Could you check a few things on this model? Use its own coordinates, in mm. A direction names the side the tool comes from. Give positions to 0.01 mm unless a question says otherwise; leave off trailing zeros. Write each loop counter-clockwise with the first axis right and the second up, starting at its lowest first coordinate (ties: lowest second). Pieces come first, ordered by that corner, then holes. Notation, with made-up numbers: (54, 64.25) -> (62, 64.25) arc R22 cw to (62, 101.25) -> close; hole circle Ø5 at (-35.5, 51.25). An arc over 180 degrees is marked (long way). One line per question, with ' | ' between items.
from build123d import *

# Parameters (mm, degrees)
SKETCH_1_R          = 1.85
EXTRUDE_1_DEPTH     = 13
SKETCH_2_R          = 2.6
CUT_EXTRUDE_1_DEPTH = 10
SKETCH_3_R          = 2.6
CUT_EXTRUDE_2_DEPTH = 10
FILLET_1_R          = 2
FILLET_2_R          = 1
SKETCH_4_R          = 3.5
SKETCH_4_R_2        = 1.85
CUT_EXTRUDE_3_DEPTH = 7
CUT_EXTRUDE_5_DEPTH = 61.729236251
CUT_EXTRUDE_START   = -4
SKETCH_6_R          = 5.5
SKETCH_6_R_2        = 2.6
CUT_EXTRUDE_6_DEPTH = 4
SKETCH_7_R          = 5.5
SKETCH_7_R_2        = 2.6
CUT_EXTRUDE_7_DEPTH = 4


with BuildPart() as part:
    # 草图1 → 凸台-拉伸1 (new body)
    with BuildSketch(Plane(origin=(0, 0, 0), x_dir=(1, 0, 0), z_dir=(0, 1, 0))):
        with BuildLine():
            ThreePointArc((-18.308849916, -29.829281164), (-22.856098901, -26.50657924), (-26.811555509, -22.497566339))
            Line((-26.811555509, -22.497566339), (-36.387111048, -30.53241146))
            ThreePointArc((-36.387111048, -30.53241146), (0, -47.5), (36.387111048, -30.53241146))
            Line((36.387111048, -30.53241146), (26.811555509, -22.497566339))
            ThreePointArc((26.811555509, -22.497566339), (22.856098901, -26.50657924), (18.308849916, -29.829281164))
            Line((18.308849916, -29.829281164), (19.814649575, -33.464603124))
            Line((19.814649575, -33.464603124), (9.651974717, -37.67412088))
            Line((9.651974717, -37.67412088), (8.146175058, -34.03879892))
            ThreePointArc((8.146175058, -34.03879892), (0, -35), (-8.146175058, -34.03879892))
            Line((-8.146175058, -34.03879892), (-9.651974717, -37.67412088))
            Line((-9.651974717, -37.67412088), (-19.814649575, -33.464603124))
            Line((-19.814649575, -33.464603124), (-18.308849916, -29.829281164))
        make_face()
        with BuildLine():
            ThreePointArc((-28.2020382, -30.0520382), (-28.237585432, -30.412955296), (-28.342861065, -30.76000255))
            ThreePointArc((-28.342861065, -30.76000255), (-31.866490969, -29.691121105), (-28.2020382, -30.0520382))
        make_face(mode=Mode.SUBTRACT)
        with BuildLine():
            ThreePointArc((1.85, -42.5), (-0.360917096, -44.314452769), (-1.709177135, -41.79203565))
            ThreePointArc((-1.709177135, -41.79203565), (0.360917096, -40.685547231), (1.85, -42.5))
        make_face(mode=Mode.SUBTRACT)
        with Locations(Location((30.0520382, -30.0520382, 0), (0, 0, 90))):
            Circle(SKETCH_1_R, mode=Mode.SUBTRACT)
    extrude(amount=EXTRUDE_1_DEPTH)

    # 草图2 → 切除-拉伸1 (cut)
    with BuildSketch(Plane(origin=(-14.733312146, 0, 35.569362002), x_dir=(-0.9238795325112864, 0, -0.38268343236509067), z_dir=(0.38268343236509067, 0, -0.9238795325112864))):
        with Locations((0, 6.5)):
            Circle(SKETCH_2_R)
    extrude(amount=-CUT_EXTRUDE_1_DEPTH, mode=Mode.SUBTRACT)

    # 草图3 → 切除-拉伸2 (cut)
    with BuildSketch(Plane(origin=(14.733312146, 0, 35.569362002), x_dir=(-0.9238795325112864, 0, 0.38268343236509067), z_dir=(-0.38268343236509067, 0, -0.9238795325112864))):
        with Locations((0, 6.5)):
            Circle(SKETCH_3_R)
    extrude(amount=-CUT_EXTRUDE_2_DEPTH, mode=Mode.SUBTRACT)

    # 圆角1
    fillet_1_edges = [part.edges().sort_by_distance(p)[0] for p in [
        (-26.811555509, 6.5, 22.497566339),
        (26.811555509, 6.5, 22.497566339),
        (36.387111048, 6.5, 30.53241146),
        (-36.387111048, 6.5, 30.53241146),
    ]]
    fillet(fillet_1_edges, radius=FILLET_1_R)

    # 圆角2
    fillet_2_edges = [part.edges().sort_by_distance(p)[0] for p in [
        (-18.308849916, 6.5, 29.829281164),
        (-8.146175058, 6.5, 34.03879892),
        (8.146175058, 6.5, 34.03879892),
        (18.308849916, 6.5, 29.829281164),
    ]]
    fillet(fillet_2_edges, radius=FILLET_2_R)

    # 草图4 → 切除-拉伸3 (cut)
    # profile 1 of 3: a face of its own
    with BuildSketch(Plane.XZ):
        with Locations(Location((-30.0520382, 30.0520382, 0), (0, 0, 270))):
            Circle(SKETCH_4_R)
        with Locations(Location((-30.0520382, 30.0520382, 0), (0, 0, 270))):
            Circle(SKETCH_4_R_2, mode=Mode.SUBTRACT)
    # profile 2 of 3: a face of its own
    with BuildSketch(Plane.XZ):
        with Locations(Location((0, 42.5, 0), (0, 0, 270))):
            Circle(SKETCH_4_R)
        with Locations(Location((0, 42.5, 0), (0, 0, 270))):
            Circle(SKETCH_4_R_2, mode=Mode.SUBTRACT)
    # profile 3 of 3: a face of its own
    with BuildSketch(Plane.XZ):
        with Locations(Location((30.0520382, 30.0520382, 0), (0, 0, 270))):
            Circle(SKETCH_4_R)
        with Locations(Location((30.0520382, 30.0520382, 0), (0, 0, 270))):
            Circle(SKETCH_4_R_2, mode=Mode.SUBTRACT)
    extrude(amount=-CUT_EXTRUDE_3_DEPTH, mode=Mode.SUBTRACT)

    # 草图5 → 切除-拉伸5 (cut, through all)
    with BuildSketch(Plane.XZ):
        with BuildLine():
            Line((-23.136534812, 41.484343515), (-18.055197383, 43.589102393))
            Line((-18.055197383, 43.589102393), (-18.177463037, 43.884277794))
            ThreePointArc((-18.177463037, 43.884277794), (-20.691822677, 42.756268246), (-23.136534812, 41.484343515))
        make_face()
        with BuildLine():
            Line((-18.177463037, 43.884277794), (-18.055197383, 43.589102393))
            Line((-18.055197383, 43.589102393), (-12.973859954, 45.693861271))
            ThreePointArc((-12.973859954, 45.693861271), (-15.601919085, 44.864575345), (-18.177463037, 43.884277794))
        make_face()
        with BuildLine():
            ThreePointArc((18.177463037, 43.884277794), (15.601919085, 44.864575345), (12.973859954, 45.693861271))
            Line((12.973859954, 45.693861271), (18.055197383, 43.589102393))
            Line((18.055197383, 43.589102393), (18.177463037, 43.884277794))
        make_face()
        with BuildLine():
            Line((18.177463037, 43.884277794), (18.055197383, 43.589102393))
            Line((18.055197383, 43.589102393), (23.136534812, 41.484343515))
            ThreePointArc((23.136534812, 41.484343515), (20.691822677, 42.756268246), (18.177463037, 43.884277794))
        make_face()
    extrude(amount=-CUT_EXTRUDE_5_DEPTH, mode=Mode.SUBTRACT)

    # 草图6 → 切除-拉伸6 (cut)
    with BuildSketch(Plane(origin=(-18.055197383, 0, 43.589102393), x_dir=(0.9238795325112865, 0, 0.38268343236509045), z_dir=(-0.38268343236509045, 0, 0.9238795325112865)).offset(CUT_EXTRUDE_START)):
        with Locations((0, 6.5)):
            Circle(SKETCH_6_R)
        with Locations(Location((0, 6.5, 0), (0, 0, 180))):
            Circle(SKETCH_6_R_2, mode=Mode.SUBTRACT)
    extrude(amount=CUT_EXTRUDE_6_DEPTH, mode=Mode.SUBTRACT)

    # 草图7 → 切除-拉伸7 (cut)
    with BuildSketch(Plane(origin=(18.055197383, 0, 43.589102393), x_dir=(0.9238795325112865, 0, -0.38268343236509045), z_dir=(0.38268343236509045, 0, 0.9238795325112865)).offset(CUT_EXTRUDE_START)):
        with Locations((0, 6.5)):
            Circle(SKETCH_7_R)
        with Locations(Location((0, 6.5, 0), (0, 0, 180))):
            Circle(SKETCH_7_R_2, mode=Mode.SUBTRACT)
    extrude(amount=CUT_EXTRUDE_7_DEPTH, mode=Mode.SUBTRACT)


solid = part.part
Q1. Imagine slicing it at A-A on x = 0. Please give me the cut outline in (y, z).
Answer below:
outline: (0, 35) -> (13, 35) -> (13, 40.65) -> (7, 40.65) -> (7, 39) -> (0, 39) -> close; (0, 46) -> (7, 46) -> (7, 44.35) -> (13, 44.35) -> (13, 47.5) -> (0, 47.5) -> close
Q2. If I drill on line 1 along X through (y, z) = (6.5, 29); line 2 along X through (y, z) = (6.25, 28); line 3 along X through (y, z) = (10, 39), over which ranges is the centre line in solid material (lowest first)?
Answer below:
line 1: x = -34.56 to -33.39, -26.71 to -19.6, 19.6 to 26.71, 33.39 to 34.56 | line 2: x = -33.37 to -32.89, -27.22 to -21, 21 to 27.22, 32.89 to 33.37 | line 3: x = -27.12 to -20.75, -18.68 to 18.68, 20.75 to 27.12
Q3. If we mould it in two halves opening along X, with no side actions, what happens to faces 5 (the flat face through (0, 13, 38)), 6 (the flat face through (-18.85, 5.35, 38.93)), 7 (the flat face through (-31.52, 6.41, 26.45))? For each: +X half, -X half, draft (parallel to the pull), parting line (faces both ways), or undercut.
Answer below:
face 5: draft | face 6: undercut | face 7: -X half
Q4. Imagine slicing it at B-B on y = 5.5. Count the separate pieces of the cut face and the enclosed holes in it, and give its area (3 significant figures).
Answer below:
separate pieces: 3 | enclosed holes: 3 | area: 564 mm^2
Q5. On a 3-axis mill with a long thin cutter (end or side, diameter ignored), from which of +Z, -Z, +X, -X, +Y, -Y can I reach the whole of each face in a straight line? I mean faces 1 (the cylindrical face through (29.366, 6.409, 37.335)), 2 (the cylindrical face through (22.5, 6.41, 26.81)), 3 (the flat face through (-12.404, 4.965, 36.534)), 4 (the flat face through (-32, 7, 29)). Say none if no direction works.
Answer below:
face 1: +Z, +X, +Y, -Y | face 2: -Z, +Y, -Y | face 3: +Y, -Y | face 4: -Y
Q6. Will these pins go through, and if not, where does the flat tip stop? pin 1 (2 mm diameter, centred on x = 1, z = 43, fed in from -Y); pin 2 (1.5 mm diameter, centred on y = 6.5, z = 39, fed in from +X); pin 3 (1 mm diameter, centred on x = -2, y = 3, fed in from +Z).
Answer below:
pin 1: stops at y = 7 | pin 2: stops at x = 28.16 | pin 3: stops at z = 47.48
